Build history of the part. All positions in model axes, mm. A direction names the side the tool comes from. Give positions to 0.01 mm unless a question says otherwise; leave off trailing zeros. Order: outer loops, then holes, each group sorted by start corner. A loop starts at its lowest first (then second) coordinate and runs counter-clockwise, first axis right, second up. Notation, with made-up numbers: (29.5, 84.5) - (61.5, 84.5) arc R28 ccw to (61.5, 108.5) - close; hole circle Ø3 at (-7, -3.75). An arc over 180 degrees is marked (long way). Answer in a Markdown table with one row per item.
Autodesk Inventor part; units mm, degrees
ref_plane "YZ Plane" through (0, 0, 0) normal (1, 0, 0) x (0, 1, 0)
ref_plane "XZ Plane" through (0, 0, 0) normal (0, 1, 0) x (-1, 0, 0)
ref_plane "XY Plane" through (0, 0, 0) normal (0, 0, 1) x (1, 0, 0)
sketch "スケッチ1" plane through (0, 0, 0) normal (0, 1, 0) x (-1, 0, 0)
  line L0 (0, 0) -> (-39, 0)
  line L1 (-39, 0) -> (-39, -54)
  line L2 (-39, -54) -> (0, -54)
  line L3 (0, -54) -> (0, 0)
  dimension "d0" = 39
  dimension "d1" = 54
extrude "押し出し1" add sketch "スケッチ1" along normal blind 1
sketch "スケッチ3" plane through (0, 1, 0) normal (0, 1, 0) x (1, 0, 0)
  line L0 (1, 1) -> (38, 1)
  line L1 (38, 1) -> (38, 54)
  line L2 (38, 54) -> (1, 54)
  line L3 (1, 54) -> (1, 1)
  line L4 (39, 54) -> (0, 54)
  line L5 (0, 54) -> (0, 0)
  dimension "d4" = 37
  dimension "d5" = 53
  dimension "d6" = 0
  dimension "d7" = 1
extrude "押し出し2" add sketch "スケッチ3" along normal blind 1
fillet "フィレット1" radius 1 1 edges at (19.5, 2, -54)
properties part number "case_top"
1. Which spindle directions (+Z, -Z, +X, -X, +Y, -Y) get a long thin tool onto all of the face, cutting with end or side? Do faces 1 (the face through (19.241, 1.715, -53.699)), 2 (the face through (19.2, 1.5, -1)), 3 (the face through (38, 1.5, -27.1)), 4 (the face through (1, 1.5, -27.9)). Say none if no direction does.
Check result:
| item | result |
|---|---|
| face 1 | -Z, +X, -X, +Y |
| face 2 | +Z, +X, -X, +Y |
| face 3 | +Z, -Z, +X, +Y |
| face 4 | +Z, -Z, -X, +Y |
2. Cut at A-A on z = -14. Write the cut outline in (x, y).
Check result:
| item | result |
|---|---|
| outline | (0, 0) - (39, 0) - (39, 1) - (38, 1) - (38, 2) - (1, 2) - (1, 1) - (0, 1) - close |
3. Probe line 1 (Z direction, x = 34, y = 1.05); line 2 (X direction, y = 1.8, z = -40.5); line 3 (Z direction, x = 37, y = 1.5). List the from-to ranges inside material, lowest first.
Check result:
| item | result |
|---|---|
| line 1 | z = -54 to -1 |
| line 2 | x = 1 to 38 |
| line 3 | z = -53.87 to -1 |
4. Drop flat-ended pins along their axis: P1, Ø0.8, axis at y = 1.5, z = -34.5, coming from the -X side; P2, Ø0.8, axis at x = 28, y = 1.5, coming from the +Z side; P3, Ø0.5, axis at y = 1.5, z = -32.5, coming from the +X side. Give the stop position or say it passes through.
Check result:
| item | result |
|---|---|
| P1 | stops at x = 1 |
| P2 | stops at z = -1 |
| P3 | stops at x = 38 |
